Work out the finished part from the listing and answer in its coordinate system (mm). Face numbers are marked on the shaded views. A direction names the side the tool comes from. Give positions to 0.01 mm unless a question says otherwise; leave off trailing zeros. Loops run counter-clockwise (first coordinate to the right, second up) from the corner with the lowest first, then second, coordinate; pieces in that order, holes last.
from build123d import *

# Parameters (mm, degrees)
F0_W      = 40
F0_H      = 100
F1_DEPTH  = 45
F2_R      = 15
F3_DEPTH  = 90
F5_DEPTH  = 45.001
F7_DEPTH  = 100.001
F9_DEPTH  = 25
F10_R     = 10
F11_DEPTH = 100.001
F14_DEPTH = 40


with BuildPart() as f1:
    # F0 (on Front) → F1 (new body)
    with BuildSketch(Plane.XZ):
        with Locations((20, 50)):
            Rectangle(F0_W, F0_H)
    extrude(amount=-F1_DEPTH)

    # F2 (on face) → F3 (join)
    with BuildSketch(Plane.XY.offset(100)):
        with Locations((40, 15)):
            Circle(F2_R)
    extrude(amount=-F3_DEPTH)

    # F4 (on face) → F5 (cut, through all)
    with BuildSketch(Plane.XZ):
        Polygon((62.4297, 100), (0, 100), (40, 80), (62.4297, 80), align=None)
    extrude(amount=-F5_DEPTH, mode=Mode.SUBTRACT)

    # F6 (on Top) → F7 (cut, through all)
    with BuildSketch(Plane.XY):
        Polygon((30, 40), (5, 40), (5, 5), (20, 5), (30, 30), align=None)
    extrude(amount=F7_DEPTH, mode=Mode.SUBTRACT)

    # F8 (on face) → F9 (join)
    with BuildSketch(Plane(origin=(0, 0, 0), x_dir=(1, 0, 0), z_dir=(0, 0, -1))):
        Polygon((5, -5), (5, -40), (30, -40), (30, -30), (20, -5), align=None)
    extrude(amount=-F9_DEPTH)

    # F10 (on Top) → F11 (cut, through all)
    with BuildSketch(Plane.XY):
        with Locations((40, 15)):
            Circle(F10_R)
    extrude(amount=F11_DEPTH, mode=Mode.SUBTRACT)

    # F13 (on offset) → F14 (join)
    with BuildSketch(Plane.XY.offset(25)):
        Polygon((20, 0), (0, 0), (0, -40), align=None)
    extrude(amount=F14_DEPTH)


solid = f1.part
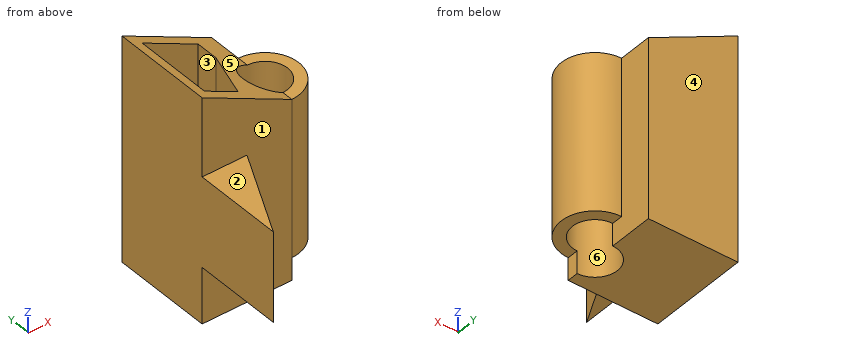
Item 1: Find section C-C, the plane y = 22. Write down the section's boundary in (x, z).
Item 2: Find section B-B, the plane z = 59. Write down the section's boundary in (x, y).
Item 3: Determine the mould class of the marked faces 4, 5 and 6 for opening direction Y: released by +Y, released by -Y, zero draft, split by the parting line, or undercut.
Item 4: Flat-ended cylindrical pins translate along their axes: pin 1 Ø2 at (y, z) = (30, 88) entering from -X; pin 2 Ø7.5 at (x, y) = (50.5, 22) entering from +Z; pin 3 Ø4 at (y, z) = (2, 3.5) entering from +X; pin 4 Ø16 at (x, y) = (5, -14.5) entering from -Z. Find the tip coordinate at first contact, or state that the pin passes through.
Item 5: Consider line 1 (X direction, y = 15, z = 68); line 2 (Y direction, x = 19.5, z = 66.5); line 3 (Z direction, x = 47.5, y = 3). Determine where each line is inside the solid, lowest interval first.
Item 6: For the marked faces 1, 2 and 3, determine the directions among +Z, -Z, +X, -X, +Y, -Y from which every point of the face is accessible in a straight line to the end or side of a thin tool.
Item 7: Find section A-A, the plane y = 31.5. Write down the section's boundary in (x, z), plus the area to 3 significant figures.
Item 8: Find section D-D, the plane x = 7. Write down the section's boundary in (y, z), plus the area to 3 significant figures.
Ans:
1. outline: (0, 0) - (32.86, 0) - (32.86, 83.57) - (26.8, 86.6) - (26.8, 25) - (5, 25) - (5, 97.5) - (0, 100) - close; (47.14, 10) - (53.27, 10) - (53.27, 80) - (47.14, 80) - close
2. outline: (0, -40) - (20, 0) - (40, 0) arc R15 ccw to (40, 30) - (40, 45) - (0, 45) - close; hole (5, 5) - (20, 5) - (30, 30) - (30, 40) - (5, 40) - close; hole circle Ø20 at (40, 15)
3. face 4: released by +Y
3. face 5: zero draft
3. face 6: undercut
4. pin 1: stops at x = 0
4. pin 2: stops at z = 80
4. pin 3: stops at x = 40
4. pin 4: stops at z = 25
5. line 1: x = 0 to 5, 24 to 30, 50 to 55
5. line 2: y = 0 to 5, 40 to 45
5. line 3: z = 10 to 80
6. face 1: +X, -Y
6. face 2: +Z, +X, -X, -Y
6. face 3: +Z
7. outline: (0, 0) - (40, 0) - (40, 80) - (30, 85) - (30, 25) - (5, 25) - (5, 97.5) - (0, 100) - close
7. area: 1,940 mm2
8. outline: (-26, 25) - (0, 25) - (0, 0) - (45, 0) - (45, 96.5) - (40, 96.5) - (40, 25) - (5, 25) - (5, 96.5) - (0, 96.5) - (0, 65) - (-26, 65) - close
8. area: 2,880 mm2
